from build123d import *

# Parameters (mm, degrees)
F0_W     = 55
F0_H     = 10
F1_DEPTH = 55
F2_R     = 16.25
F3_DEPTH = 25
F4_W     = 55
F4_H     = 30
F5_DEPTH = 5
F6_R     = 2
F7_DEPTH = 25


with BuildPart() as f1:
    # F0 (on Top) → F1 (new body)
    with BuildSketch(Plane.XY):
        Rectangle(F0_W, F0_H)
    extrude(amount=F1_DEPTH)

    # F2 (on face) → F3 (cut)
    with BuildSketch(Plane.XZ.offset(5)):
        with Locations((0, 27.5)):
            Circle(F2_R)
    extrude(amount=-F3_DEPTH, mode=Mode.SUBTRACT)

    # F4 (on Top) → F5 (join)
    with BuildSketch(Plane.XY):
        Rectangle(F4_W, F4_H)
    extrude(amount=-F5_DEPTH)

    # F6 (on face) → F7 (cut)
    with BuildSketch(Plane(origin=(0, 0, -5), x_dir=(1, 0, 0), z_dir=(0, 0, -1))):
        with Locations((23.685403, 10.313298)):
            Circle(F6_R)
        with Locations((-23.685403, 10.313298)):
            Circle(F6_R)
        with Locations((-23.685403, -10.313298)):
            Circle(F6_R)
        with Locations((23.685403, -10.313298)):
            Circle(F6_R)
    extrude(amount=-F7_DEPTH, mode=Mode.SUBTRACT)


solid = f1.part
Can you work these out from the model? Positions are in its coordinate system, mm. A direction names the side the tool comes from. Coordinates: 2 decimals unless noted, no trailing zeros. Write each loop counter-clockwise with the first axis right and the second up, starting at its lowest first coordinate (ties: lowest second). Pieces come first, ordered by that corner, then holes.
Q1. If we mould it in two halves opening along Y, with no side actions, what happens to faces 4 (the face through (-13, 5, 15)), 5 (the face through (27.5, 0, 19)), 6 (the face through (0, -15, -2)), 7 (the face through (22.211, -11.665, -2.535))? For each: +Y half, -Y half, draft (parallel to the pull), parting line (faces both ways), or undercut.
Results found:
face 4: +Y half
face 5: draft
face 6: -Y half
face 7: undercut
Q2. For P1, Ø12, axis at x = 18, z = 12, coming from the +Y side; P2, Ø2.5, axis at x = 23.69, y = -10.31, coming from the +Z side; P3, Ø10, axis at y = -5.5, z = 9, coming from the -X side; P4, Ø4.5, axis at x = -23.69, y = 10.31, coming from the +Z side, each with a flat end and sliding along its axis, tell me the tip position at first contact or that it passes through.
Results found:
P1: stops at y = 5
P2: passes through
P3: stops at x = -27.5
P4: stops at z = 0
Q3. Imagine slicing it at C-C, the plane y = -11.5. List the corners of the cut face in (x, z) for me.
Results found:
outline: (-27.5, -5) - (-25.3, -5) - (-25.3, 0) - (-27.5, 0) - close; (-22.08, -5) - (22.08, -5) - (22.08, 0) - (-22.08, 0) - close; (25.3, -5) - (27.5, -5) - (27.5, 0) - (25.3, 0) - close
Q4. Imagine slicing it at B-B, the plane z = 27.5. List the corners of the cut face in (x, y) for me.
Results found:
outline: (-27.5, -5) - (-16.25, -5) - (-16.25, 5) - (-27.5, 5) - close; (16.25, -5) - (27.5, -5) - (27.5, 5) - (16.25, 5) - close
Q5. Imagine slicing it at D-D, the plane y = 3.75. List the corners of the cut face in (x, z) for me, plus the area to 3 significant figures.
Results found:
outline: (-27.5, -5) - (27.5, -5) - (27.5, 55) - (-27.5, 55) - close; hole circle Ø32.5 at (0, 27.5)
area: 2,470 mm2
Q6. Imagine slicing it at A-A, the plane x = 0. List the corners of the cut face in (y, z) for me, plus the area to 3 significant figures.
Results found:
outline: (-15, -5) - (15, -5) - (15, 0) - (5, 0) - (5, 11.25) - (-5, 11.25) - (-5, 0) - (-15, 0) - close; (-5, 43.75) - (5, 43.75) - (5, 55) - (-5, 55) - close
area: 375 mm2
Q7. Which directions (+Z, -Z, +X, -X, +Y, -Y) give clear straight access to the entire face, cutting with the end or side of a thin tool? Please do faces 1 (the face through (22.1, 11.53, -2.54)), 2 (the face through (-13, -5, 15)), 3 (the face through (0, 10, 0)).
Results found:
face 1: +Z, -Z
face 2: +Z, +X, -X, -Y
face 3: +Z, +X, -X, +Y
Q8. Please list where these lines run through material, in increasing order: L1, parallel to Z at x = 0.5, y = 8.5; L2, parallel to Y at x = 25.5, z = 41.5; L3, parallel to Z at x = 10.5, y = 1.75.
Results found:
L1: z = -5 to 0
L2: y = -5 to 5
L3: z = -5 to 15.1, 39.9 to 55
